Autodesk Inventor part; units mm, degrees
ref_plane "Work Plane1" through (0, 0, 0) normal (0, 0, 1) x (1, 0, 0)
ref_plane "YZ Plane" through (0, 0, 0) normal (1, 0, 0) x (0, 1, 0)
ref_plane "XZ Plane" through (0, 0, 0) normal (0, 1, 0) x (-1, 0, 0)
ref_plane "Work Plane1" through (0, 0, 0) normal (0, 0, 1) x (1, 0, 0)
sketch "Sketch1" plane through (0, 0, 0) normal (0, 0, 1) x (1, 0, 0)
  line L0 (143.35, -48.1) -> (143.35, 29.05)
  line L1 (143.35, 29.05) -> (114.775, 29.05)
  line L2 (114.775, 29.05) -> (114.775, 48.1)
  line L3 (114.775, 48.1) -> (-95.725, 48.1)
  line L4 (-95.725, 48.1) -> (-95.725, 29.05)
  line L5 (-95.725, 29.05) -> (-143.35, 29.05)
  line L6 (-143.35, 29.05) -> (-143.35, -48.1)
  line L7 (-143.35, -48.1) -> (143.35, -48.1)
  line L8 (147.35, -58.1) -> (-147.35, -58.1)
  line L9 (-147.35, -58.1) -> (-147.35, 58.1)
  line L10 (-147.35, 58.1) -> (147.35, 58.1)
  line L11 (147.35, 58.1) -> (147.35, -58.1)
  line L12 (140.35, -31.6) -> (140.35, -44.6)
  line L13 (139.85, -45.1) -> (126.85, -45.1)
  line L14 (-140.35, -44.6) -> (-140.35, -31.6)
  line L15 (-92.725, 31.6) -> (-92.725, 44.6)
  line L16 (111.775, 44.6) -> (111.775, 31.6)
  line L17 (98.275, 45.1) -> (111.275, 45.1)
  line L18 (114.9437, 26.05) -> (127.9437, 26.05)
  point P0 (0, 0)
extrude "Extrusion1" add sketch "Sketch1" along normal blind 7.8
sketch "Sketch2" plane through (-147.35, -58.1, 0) normal (-1, 0, 0) x (0, 0, 1)
  line L0 (0, 116.2) -> (0, 0)
  line L1 (0, 116.2) -> (-11.364, 116.2)
  line L2 (0, 116.2) -> (7.8, 116.2)
  line L3 (-11.364, 116.2) -> (-14.6271, 91.4139)
  arc A0 (-14.6271, 91.4139) -> (-13.5342, 45.2415) centre (134.0896, 71.8349) ccw
  arc A1 (-11.9235, 3.5135) -> (-13.5342, 45.2415) centre (-161.158, 18.648) ccw
  arc A2 (-11.9235, 3.5135) -> (-12, 2) centre (3, 2) ccw
  line L4 (-12, 2) -> (-12, 0)
  line L5 (0, 0) -> (-12, 0)
  line L6 (0, 0) -> (7.8, 0)
  line L7 (-11.364, 116.2) -> (-11.0375, 118.68) construction
  line L8 (7.8, 116.2) -> (-11.0375, 118.68) construction
  point P0 (0, 58.1)
  dimension "d14" = 97.5
  dimension "d15" = 25
  dimension "d16" = 150
  dimension "d17" = 150
  dimension "d18" = 2
  dimension "d19" = 15
  dimension "d22" = 12
  dimension "d34" = 19
  dimension "d35" = 19.1639
extrude "Extrusion2" add sketch "Sketch2" against normal blind 2
mirror "Mirror1" about plane through (0, 0, 0) normal (1, 0, 0) of "Extrusion2"
sketch "Sketch3" plane through (0, 0, 0) normal (0, 0, -1) x (-1, 0, 0)
  line L0 (-145.35, 58.1) -> (145.35, 58.1)
  line L1 (145.35, -58.1) -> (-145.35, -58.1)
  line L2 (145.35, -58.1) -> (145.35, 58.1)
  line L3 (-145.35, 58.1) -> (-145.35, -58.1)
  line L4 (145.35, 56.1) -> (-145.35, 56.1)
  line L5 (145.35, -56.1) -> (-145.35, -56.1)
  point P0 (0, 0)
  dimension "d25" = 2
  dimension "d26" = 2
extrude "Extrusion3" add sketch "Sketch3" along normal up to surface contours L0 L2 L4 L3 surface through (-147.35, 33.3139, -14.6271) normal (0, 0.1305, -0.9914)
sketch "Sketch4" plane through (-147.35, -58.1, 7.8) normal (0, -1, 0) x (1, 0, 0)
  line L0 (2, -7.8) -> (2, -19.8)
  line L1 (2, -7.8) -> (292.7, -7.8)
  line L2 (292.7, -7.8) -> (292.7, -19.8)
  line L3 (0, -19.8) -> (2, -19.8)
  line L4 (294.7, -19.8) -> (292.7, -19.8)
  arc A0 (2, -19.8) -> (2.542, -19.7902) centre (2, -4.8) ccw
  arc A1 (147.35, -19.8) -> (2.542, -19.7902) centre (74.8108, -2018.4841) ccw
  arc A2 (147.35, -19.8) -> (292.158, -19.8098) centre (219.8892, 1978.8841) ccw
  arc A3 (292.7, -19.8) -> (292.158, -19.8098) centre (292.7, -34.8) ccw
  point P0 (147.35, -7.8)
  point P1 (147.35, -7.8)
  dimension "d29" = 15
  dimension "d30" = 2000
  dimension "d36" = 2000
extrude "Extrusion4" add sketch "Sketch4" against normal blind 2
properties part number "top"
Geometry: final body of the model. Coordinates: model frame, mm. A direction names the side the tool comes from. Round coordinates to 2 decimals unless told otherwise and drop trailing zeros. Order: outer loops, then holes, each group sorted by start corner. A loop starts at its lowest first (then second) coordinate and runs counter-clockwise, first axis right, second up.
Q1. Section A-A, the plane z = -8. Output: boundary loops of the cut face in (x, y).
Result sheet:
outline: (-147.35, -58.1) - (147.35, -58.1) - (147.35, 58.1) - (-147.35, 58.1) - close; hole (-145.35, -56.1) - (145.35, -56.1) - (145.35, 56.1) - (-145.35, 56.1) - close
Q2. Section B-B, the plane x = 53.5. Output: boundary loops of the cut face in (y, z), and give its area (3 significant figures).
Result sheet:
outline: (-58.1, -13.23) - (-56.1, -13.23) - (-56.1, 0) - (-48.1, 0) - (-48.1, 7.8) - (-58.1, 7.8) - close; (48.1, 0) - (56.1, 0) - (56.1, -11.63) - (58.1, -11.36) - (58.1, 7.8) - (48.1, 7.8) - close
area: 205 mm2
Q3. Section D-D, the plane z = 3.25. Output: boundary loops of the cut face in (x, y) (3 decimals).
Result sheet:
outline: (-147.35, -58.1) - (147.35, -58.1) - (147.35, 58.1) - (-147.35, 58.1) - close; hole (-143.35, -48.1) - (143.35, -48.1) - (143.35, 29.05) - (114.775, 29.05) - (114.775, 48.1) - (-95.725, 48.1) - (-95.725, 29.05) - (-143.35, 29.05) - close
Q4. Pin query (flat end, axial travel): pin 1 (0.6 mm diameter, centred on x = 146.5, y = -57, fed in from -Z). Return the tip coordinate at first contact, or that it passes through.
Result sheet:
pin 1: stops at z = -12
Q5. Access query for faces 1 (the face through (147.35, 1, -4)), 2 (the face through (-11, 50, 0)), 3 (the face through (129, 29.05, 4)). Directions: +Z, -Z, +X, -X, +Y, -Y. A direction counts if a zero-diameter tool reaches every point of the face in a straight line with its end or side. Return the directions, or none.
Result sheet:
face 1: +Z, -Z, +X, +Y, -Y
face 2: -Z
face 3: +Z, -Z
Q6. Section C-C, the plane y = 25.5. Output: boundary loops of the cut face in (x, z).
Result sheet:
outline: (-147.35, -15.45) - (-145.35, -15.45) - (-145.35, 0) - (-143.35, 0) - (-143.35, 7.8) - (-147.35, 7.8) - close; (143.35, 0) - (145.35, 0) - (145.35, -15.45) - (147.35, -15.45) - (147.35, 7.8) - (143.35, 7.8) - close
Q7. Mould query, pull axis Y, two halves, no side actions, for faces 4 (the face through (-2, -48.1, 4)), 5 (the face through (-2, -58.1, -3)), 6 (the face through (2, 58.1, -2)). Classes: released by +Y, released by -Y, zero draft, split by the parting line, or undercut.
Result sheet:
face 4: undercut
face 5: released by -Y
face 6: released by +Y
Q8. Material intervals for probe 1 along Y at (x, z) = (-7.5, -7); probe 2 along X at (y, z) = (15, -10); probe 3 along X at (y, z) = (13.5, 5.75), sorted ascending.
Result sheet:
probe 1: y = -58.1 to -56.1, 56.1 to 58.1
probe 2: x = -147.35 to -145.35, 145.35 to 147.35
probe 3: x = -147.35 to -143.35, 143.35 to 147.35
